from build123d import *

# Parameters (mm, degrees)
SKETCH1_R                                          = 50.8
SKETCH1_R_2                                        = 6.35
BOSS_EXTRUDE1_DEPTH                                = 6.35
CUT_EXTRUDE1_DEPTH                                 = 6.35
CIRPATTERN1_COUNT                                  = 32
CSK_FOR_10_FLAT_HEAD_MACHINE_SCREW_100_D           = 5.1054
CSK_FOR_10_FLAT_HEAD_MACHINE_SCREW_100_CSINK_D     = 9.779
CSK_FOR_10_FLAT_HEAD_MACHINE_SCREW_100_CSINK_ANGLE = 100
CIRPATTERN2_COUNT                                  = 4


with BuildPart() as part:
    # Sketch1 → Boss-Extrude1 (new body)
    with BuildSketch(Plane(origin=(0, 0, 0), x_dir=(1, 0, 0), z_dir=(0, 1, 0))):
        with Locations(Location((0, 0, 0), (0, 0, 270))):
            Circle(SKETCH1_R)
        with Locations(Location((0, 0, 0), (0, 0, 270))):
            Circle(SKETCH1_R_2, mode=Mode.SUBTRACT)
    extrude(amount=BOSS_EXTRUDE1_DEPTH)

    # Sketch2 → Cut-Extrude1 (cut)
    with BuildSketch(Plane.XY.offset(50.8)):
        Polygon((-11.786586159, 18.329182204), (15.154182204, -8.611586159), (11.786586159, -11.979182204), (-15.154182204, 14.961586159), align=None)
    cut_extrude1 = extrude(amount=-CUT_EXTRUDE1_DEPTH, mode=Mode.SUBTRACT)

    # CirPattern1: Cut-Extrude1 ×32 about axis
    cirpattern1_axis = Axis((0, 0, 0), (0, 1, 0))
    for i in range(1, CIRPATTERN1_COUNT):
        add(cut_extrude1.rotate(cirpattern1_axis, i * 360 / CIRPATTERN1_COUNT), mode=Mode.SUBTRACT)

    # CSK for #10 Flat Head Machine Screw (100)1 (through all)
    with Locations(Plane(origin=(0, 0, 31.75), x_dir=(0, 0, -1), z_dir=(0, -1, 0))):
        with Locations((0, 0)):
            csk_for_10_flat_head_machine_screw_100 = CounterSinkHole(CSK_FOR_10_FLAT_HEAD_MACHINE_SCREW_100_D / 2, CSK_FOR_10_FLAT_HEAD_MACHINE_SCREW_100_CSINK_D / 2, counter_sink_angle=CSK_FOR_10_FLAT_HEAD_MACHINE_SCREW_100_CSINK_ANGLE)

    # CirPattern2: CSK for #10 Flat Head Machine Screw (100)1 ×4 about axis
    cirpattern2_axis = Axis((0, 0, 0), (0, 1, 0))
    for i in range(1, CIRPATTERN2_COUNT):
        add(csk_for_10_flat_head_machine_screw_100.rotate(cirpattern2_axis, i * 360 / CIRPATTERN2_COUNT), mode=Mode.SUBTRACT)


solid = part.part
The model under review builds one solid part; all positions refer to its coordinate system, in mm. A direction names the side the tool comes from. Give positions to 0.01 mm unless a question says otherwise; leave off trailing zeros. Put each result on its own line as item: value. Start each with the question number.
1. Mouldability with a two-part tool opening along X and no side actions: class faces 5 (the face through (-5.002, 3.16, 50.553)), 6 (the face through (37.789, 3.131, 29.247)), 7 (the face through (0.767, 4.186, 34.185)) as released by +X, released by -X, zero draft, split by the parting line, or undercut.
2. We need section A-A on y = 4.5. State how many separate pieces and enclosed holes the cut face has, then the cut area to 3 significant figures.
3. Wall thickness on probe 1 along Z at (x, y) = (-31.75, 2.9); probe 2 along Z at (x, y) = (38.5, 5.5); probe 3 along X at (y, z) = (4.6, 31.75): over which ranges is each line inside the solid? List them lowest first.
4. Clearance check with flat-ended pins moving along their axes: P1, Ø3, axis at y = 3.5, z = 3, coming from the -X side; P2, Ø2, axis at x = 13, y = 4, coming from the -Z side; P3, Ø1, axis at x = -28.5, y = 4.5, coming from the +Z side. State where each tip first meets the part, or that it passes through.
5. For faces 1 (the face through (-21.31, 3.22, -42.77)), 2 (the face through (23.72, 3.22, -41.48)), 3 (the face through (24.77, 3.22, 36.91)), 4 (the face through (-41.48, 3.13, 23.72)), list the 3-axis set-ups (+Z, -Z, +X, -X, +Y, -Y) from which the entire face can be reached by the end or side of a thin tool; tool diameter is ignored.
Determined:
1. face 5: released by -X
1. face 6: released by +X
1. face 7: undercut
2. separate pieces: 1
2. enclosed holes: 5
2. area: 6,540 mm^2
3. probe 1: -39.66 to -36.12, -31.11 to -2.55, 2.55 to 31.11, 36.9 to 39.66
3. probe 2: -30.45 to -26.98, -22.39 to 24.47, 32.57 to 33.14
3. probe 3: -39.66 to -38.53, -31.11 to -2.55, 2.55 to 31.11, 34.5 to 38.89
4. P1: x = -50.76
4. P2: z = -49.1
4. P3: z = 35.38
5. face 1: -Z, -Y
5. face 2: -Y
5. face 3: none
5. face 4: +Y
